Geometry check sheet. Reference: the model listing, model coordinates, mm. A direction names the side the tool comes from. Round coordinates to 2 decimals unless told otherwise and drop trailing zeros. Loops run counter-clockwise (first coordinate to the right, second up) from the corner with the lowest first, then second, coordinate; pieces in that order, holes last. Notation, with made-up numbers: (-0.75, 53.5) - (39.25, 53.5) arc R13 cw to (39.25, 64.5) - close; hole circle Ø11 at (44, -32). An arc over 180 degrees is marked (long way). Write item = value, one per line.
```python
from build123d import *

# Parameters (mm, degrees)
EXTRUDE_1_DEPTH = 50
EXTRUDE_2_DEPTH = 10


with BuildPart() as part:
    # 草图1 → 凸台-拉伸1 (new, symmetric)
    with BuildSketch(Plane.XY):
        with BuildLine():
            Line((-3.646611731, 20.680962813), (-3.993908086, 22.650578319))
            ThreePointArc((-3.993908086, 22.650578319), (-23, 0), (-3.993908086, -22.650578319))
            Line((-3.993908086, -22.650578319), (-3.646611731, -20.680962813))
            ThreePointArc((-3.646611731, -20.680962813), (-21, 0), (-3.646611731, 20.680962813))
        make_face()
    extrude(amount=EXTRUDE_1_DEPTH, both=True)

    # 草图2 → 凸台-拉伸2 (add, symmetric)
    with BuildSketch(Plane.XY):
        with BuildLine():
            Line((-3.993908086, 22.650578319), (-20.254671357, 22.911623668))
            Line((-20.254671357, 22.911623668), (-20.254671357, 20.911623668))
            Line((-20.254671357, 20.911623668), (-9.930184633, 20.745877498))
            ThreePointArc((-9.930184633, 20.745877498), (-7.026881301, 21.900295413), (-3.993908086, 22.650578319))
        make_face()
    extrude(amount=EXTRUDE_2_DEPTH, both=True)


solid = part.part
```
(1) Gauge pin test, flat ends, axial feed: pin 1 (10 mm diameter, centred on y = -1.5, z = -39.5, fed in from +X); pin 2 (6 mm diameter, centred on x = -12.5, z = 9, fed in from +Y); pin 3 (8 mm diameter, centred on y = -8, z = -21.5, fed in from -X). Record the tip position at first contact, or that the pin passes through.
Answers follow:
pin_1 = -19.97
pin_2 = 22.84
pin_3 = -22.65
(2) Section check A-A (x = -15.5). Enter the section's corners in (y, z).
Answers follow:
outline = (-16.99, -50) - (-14.17, -50) - (-14.17, 50) - (-16.99, 50) - close; (14.17, -50) - (16.99, -50) - (16.99, 50) - (14.17, 50) - close; (20.84, -10) - (22.84, -10) - (22.84, 10) - (20.84, 10) - close
(3) Scan lines: L1, parallel to Y at x = -12.5, z = -1; L2, parallel to Y at x = -8, z = 41.5; L3, parallel to Y at x = -10.75, z = -3.5. Record each from-to range of solid material in increasing order. Write a range as [from, to].
Answers follow:
L1 = [-19.31, -16.87], [16.87, 19.31], [20.79, 22.79]
L2 = [-21.56, -19.42], [19.42, 21.56]
L3 = [-20.33, -18.04], [18.04, 20.33], [20.76, 22.76]
(4) Section check C-C (x = -7.5). Enter the section's corners in (y, z).
Answers follow:
outline = (-21.74, -50) - (-19.62, -50) - (-19.62, 50) - (-21.74, 50) - close; (19.62, -50) - (21.74, -50) - (21.74, -10) - (22.71, -10) - (22.71, 10) - (21.74, 10) - (21.74, 50) - (19.62, 50) - close
(5) Section check D-D (y = -18). Enter the section's corners in (x, z).
Answers follow:
outline = (-14.32, -50) - (-10.82, -50) - (-10.82, 50) - (-14.32, 50) - close
(6) Mould release check, pull along Y, two halves, no side actions. Record for faces 1 (the flat face through (-3.818, 21.652, 0.7)), 2 (the flat face through (-3.823, -21.68, 0.7)), 3 (the cylindrical face through (-21, 0, 1)), 4 (the flat face through (-14, 22, 10)): pulls with the +Y half, pulls with the -Y half, needs draft (parallel to the pull), parting line crosses it, or undercut.
Answers follow:
face_1 = pulls with the +Y half
face_2 = pulls with the -Y half
face_3 = undercut
face_4 = needs draft
(7) Section check B-B (z = 3). Enter the section's corners in (x, y), then the cut area to 3 significant figures.
Answers follow:
outline = (-20.25, 20.91) - (-9.93, 20.75) arc R23 ccw to (-3.99, -22.65) - (-3.65, -20.68) arc R21 cw to (-3.65, 20.68) - (-3.99, 22.65) - (-20.25, 22.91) - close
area = 149 mm²
(8) Set-up check for faces 5 (the flat face through (-20.255, 22, 0)), 6 (the flat face through (-14, 22, -10)), 7 (the flat face through (-21.3, 0.1, -50)): record each of +Z, -Z, +X, -X, +Y, -Y from which the full face is reachable in a straight line by a thin tool's end or side.
Answers follow:
face_5 = +Z, -Z, -X, +Y
face_6 = -Z, -X, +Y
face_7 = -Z, +X, -X, +Y, -Y
